Geometry check sheet. Reference: the model listing, model coordinates, mm. Coordinates: 2 decimals unless noted, no trailing zeros. Write each loop counter-clockwise with the first axis right and the second up, starting at its lowest first coordinate (ties: lowest second). Pieces come first, ordered by that corner, then holes. Notation, with made-up numbers: (-10.75, 88) -> (9.25, 88) arc R17 cw to (9.25, 118) -> close; hole circle Ø4 at (-33, 84.5). An arc over 180 degrees is marked (long way). Use a Markdown table: item, result.
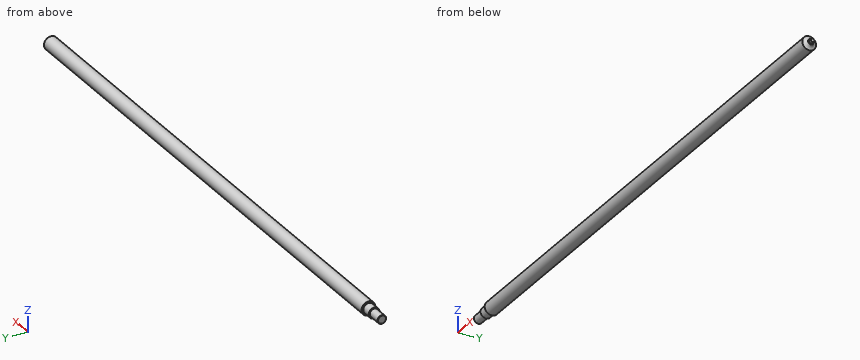
```python
from build123d import *

# Parameters (mm, degrees)
F2_SIZE = 1
F3_SIZE = 0.25
F4_SIZE = 1


with BuildPart() as f1:
    # F0 (on Front) → F1 (revolve)
    with BuildSketch(Plane.XZ):
        with BuildLine():
            Line((-39.6347922059, 59.4147157063), (-39.6347922059, 49.4147157063))
            Line((-39.6347922059, 49.4147157063), (1315.9418255951, 49.4147157063))
            Line((1315.9418255951, 49.4147157063), (1315.9418255951, 53.4147157063))
            Line((1315.9418255951, 53.4147157063), (1308.9418255951, 53.4147157063))
            Line((1308.9418255951, 53.4147157063), (1308.9418255951, 55.9769750426))
            ThreePointArc((1308.9418255951, 55.9769750426), (1303.814166428, 59.5216123442), (1301.782252331, 65.4147157063))
            Line((1301.782252331, 65.4147157063), (14.3652077941, 65.4147157063))
            Line((14.3652077941, 65.4147157063), (14.3652077941, 61.9147157063))
            Line((14.3652077941, 61.9147157063), (-7.6347922059, 61.9147157063))
            Line((-7.6347922059, 61.9147157063), (-7.6347922059, 59.4147157063))
            Line((-7.6347922059, 59.4147157063), (-39.6347922059, 59.4147157063))
        make_face()
    revolve(axis=Axis((638.1535166946, 0, 49.4147157063), (1, 0, 0)))

    # F2
    f2_edges = [f1.edges().sort_by_distance(p)[0] for p in [
        (14.365208, 0, 33.414716),
    ]]
    chamfer(f2_edges, length=F2_SIZE)

    # F3
    f3_edges = [f1.edges().sort_by_distance(p)[0] for p in [
        (-7.634792, 0, 36.914716),
    ]]
    chamfer(f3_edges, length=F3_SIZE)

    # F4
    f4_edges = [f1.edges().sort_by_distance(p)[0] for p in [
        (-39.634792, 0, 39.414716),
    ]]
    chamfer(f4_edges, length=F4_SIZE)


solid = f1.part
```
Item 1: Depth check by flat-ended pin: P1, Ø4, axis at x = 174, y = 7, coming from the +Z side; P2, Ø1, axis at y = 8, z = 42, coming from the +X side; P3, Ø1, axis at x = 275, z = 56.5, coming from the -Y side. Enter the tip coordinate at first touch or a pass-through.
Answer block:
| item | result |
|---|---|
| P1 | stops at z = 64.61 |
| P2 | stops at x = 1303.59 |
| P3 | stops at y = -14.58 |
Item 2: Section check A-A on x = 179.5. Record the boundary of the cut face in (y, z), then the cut area to 3 significant figures.
Answer block:
| item | result |
|---|---|
| outline | circle Ø32 at (0, 49.41) |
| area | 804 mm^2 |
Item 3: Thickness scan on L1, parallel to X at y = -11.5, z = 40.5; L2, parallel to Y at x = 433.5, z = 47; L3, parallel to Y at x = 290.5, z = 46.5. Record the ranges inside material, lowest first. Write a range as [from, to].
Answer block:
| item | result |
|---|---|
| L1 | x = [14.37, 1301.91] |
| L2 | y = [-15.82, 15.82] |
| L3 | y = [-15.73, 15.73] |
